Part model, mm, in its own coordinate system. Give positions to 0.01 mm unless a question says otherwise; leave off trailing zeros. Write item = value, one per line. Start each with the question number.
(1) Saw through at A-A, the plane y = 1.5. State how many separate pieces and enclosed holes the cut face has, then the cut area to 3 significant figures.
(2) Flat gauge pin, fed straight in: pin 1 (3 mm diameter, centred on x = 55.91, z = -55.35, fed in from -Y). Where does the tip first touch, or does it go through?
(3) Probe line 1 along X through (y, z) = (1.5, -90.5); line 2 along X through (y, z) = (0.25, 79.5). List the from-to ranges inside material, lowest first. Write a range as from..to.
from build123d import *

# Parameters (mm, degrees)
SKETCH1_W           = 482.6
SKETCH1_H           = 254
BOSS_EXTRUDE1_DEPTH = 3.175
FILLET1_R           = 6.35
CUT_EXTRUDE1_REACH  = 274.754
SKETCH3_R           = 3.05
CUT_EXTRUDE2_DEPTH  = 273.754491255
SKETCH4_R           = 2.5
CUT_EXTRUDE3_DEPTH  = 10


with BuildPart() as part:
    # Sketch1 → Boss-Extrude1 (new, symmetric)
    with BuildSketch(Plane(origin=(0, 0, 0), x_dir=(1, 0, 0), z_dir=(0, 1, 0))):
        Rectangle(SKETCH1_W, SKETCH1_H)
    extrude(amount=BOSS_EXTRUDE1_DEPTH, both=True)

    # Fillet1
    fillet1_edges = [part.edges().sort_by_distance(p)[0] for p in [
        (241.3, 0, 127),
        (-241.3, 0, 127),
        (-241.3, 0, -127),
        (241.3, 0, -127),
    ]]
    fillet(fillet1_edges, radius=FILLET1_R)

    # Sketch2 → Cut-Extrude1 (cut, up to next)
    with BuildSketch(Plane(origin=(0, 3.175, 0), x_dir=(1, 0, 0), z_dir=(0, 1, 0)), mode=Mode.PRIVATE) as cut_extrude1_sk1:
        with BuildLine():
            Line((227.25, -82.55), (227.25, -107.95))
            ThreePointArc((227.25, -107.95), (222.25, -112.95), (217.25, -107.95))
            Line((217.25, -107.95), (217.25, -82.55))
            ThreePointArc((217.25, -82.55), (222.25, -77.55), (227.25, -82.55))
        make_face()
    cut_extrude1_tool1 = extrude(cut_extrude1_sk1.sketch, amount=-CUT_EXTRUDE1_REACH, mode=Mode.PRIVATE) & part.part
    # Sketch2 → Cut-Extrude1 (cut, up to next)
    with BuildSketch(Plane(origin=(0, 3.175, 0), x_dir=(1, 0, 0), z_dir=(0, 1, 0)), mode=Mode.PRIVATE) as cut_extrude1_sk2:
        with BuildLine():
            Line((227.25, -44.45), (227.25, -19.05))
            ThreePointArc((227.25, -19.05), (222.25, -14.05), (217.25, -19.05))
            Line((217.25, -19.05), (217.25, -44.45))
            ThreePointArc((217.25, -44.45), (222.25, -49.45), (227.25, -44.45))
        make_face()
    cut_extrude1_tool2 = extrude(cut_extrude1_sk2.sketch, amount=-CUT_EXTRUDE1_REACH, mode=Mode.PRIVATE) & part.part
    # Sketch2 → Cut-Extrude1 (cut, up to next)
    with BuildSketch(Plane(origin=(0, 3.175, 0), x_dir=(1, 0, 0), z_dir=(0, 1, 0)), mode=Mode.PRIVATE) as cut_extrude1_sk3:
        with BuildLine():
            Line((227.25, 44.45), (227.25, 19.05))
            ThreePointArc((227.25, 19.05), (222.25, 14.05), (217.25, 19.05))
            Line((217.25, 19.05), (217.25, 44.45))
            ThreePointArc((217.25, 44.45), (222.25, 49.45), (227.25, 44.45))
        make_face()
    cut_extrude1_tool3 = extrude(cut_extrude1_sk3.sketch, amount=-CUT_EXTRUDE1_REACH, mode=Mode.PRIVATE) & part.part
    # Sketch2 → Cut-Extrude1 (cut, up to next)
    with BuildSketch(Plane(origin=(0, 3.175, 0), x_dir=(1, 0, 0), z_dir=(0, 1, 0)), mode=Mode.PRIVATE) as cut_extrude1_sk4:
        with BuildLine():
            Line((227.25, 82.55), (227.25, 107.95))
            ThreePointArc((227.25, 107.95), (222.25, 112.95), (217.25, 107.95))
            Line((217.25, 107.95), (217.25, 82.55))
            ThreePointArc((217.25, 82.55), (222.25, 77.55), (227.25, 82.55))
        make_face()
    cut_extrude1_tool4 = extrude(cut_extrude1_sk4.sketch, amount=-CUT_EXTRUDE1_REACH, mode=Mode.PRIVATE) & part.part
    # Sketch2 → Cut-Extrude1 (cut, up to next)
    with BuildSketch(Plane(origin=(0, 3.175, 0), x_dir=(1, 0, 0), z_dir=(0, 1, 0)), mode=Mode.PRIVATE) as cut_extrude1_sk5:
        with BuildLine():
            Line((-227.25, 82.55), (-227.25, 107.95))
            ThreePointArc((-227.25, 107.95), (-222.25, 112.95), (-217.25, 107.95))
            Line((-217.25, 107.95), (-217.25, 82.55))
            ThreePointArc((-217.25, 82.55), (-222.25, 77.55), (-227.25, 82.55))
        make_face()
    cut_extrude1_tool5 = extrude(cut_extrude1_sk5.sketch, amount=-CUT_EXTRUDE1_REACH, mode=Mode.PRIVATE) & part.part
    # Sketch2 → Cut-Extrude1 (cut, up to next)
    with BuildSketch(Plane(origin=(0, 3.175, 0), x_dir=(1, 0, 0), z_dir=(0, 1, 0)), mode=Mode.PRIVATE) as cut_extrude1_sk6:
        with BuildLine():
            Line((-227.25, 44.45), (-227.25, 19.05))
            ThreePointArc((-227.25, 19.05), (-222.25, 14.05), (-217.25, 19.05))
            Line((-217.25, 19.05), (-217.25, 44.45))
            ThreePointArc((-217.25, 44.45), (-222.25, 49.45), (-227.25, 44.45))
        make_face()
    cut_extrude1_tool6 = extrude(cut_extrude1_sk6.sketch, amount=-CUT_EXTRUDE1_REACH, mode=Mode.PRIVATE) & part.part
    # Sketch2 → Cut-Extrude1 (cut, up to next)
    with BuildSketch(Plane(origin=(0, 3.175, 0), x_dir=(1, 0, 0), z_dir=(0, 1, 0)), mode=Mode.PRIVATE) as cut_extrude1_sk7:
        with BuildLine():
            Line((-227.25, -44.45), (-227.25, -19.05))
            ThreePointArc((-227.25, -19.05), (-222.25, -14.05), (-217.25, -19.05))
            Line((-217.25, -19.05), (-217.25, -44.45))
            ThreePointArc((-217.25, -44.45), (-222.25, -49.45), (-227.25, -44.45))
        make_face()
    cut_extrude1_tool7 = extrude(cut_extrude1_sk7.sketch, amount=-CUT_EXTRUDE1_REACH, mode=Mode.PRIVATE) & part.part
    # Sketch2 → Cut-Extrude1 (cut, up to next)
    with BuildSketch(Plane(origin=(0, 3.175, 0), x_dir=(1, 0, 0), z_dir=(0, 1, 0)), mode=Mode.PRIVATE) as cut_extrude1_sk8:
        with BuildLine():
            Line((-227.25, -82.55), (-227.25, -107.95))
            ThreePointArc((-227.25, -107.95), (-222.25, -112.95), (-217.25, -107.95))
            Line((-217.25, -107.95), (-217.25, -82.55))
            ThreePointArc((-217.25, -82.55), (-222.25, -77.55), (-227.25, -82.55))
        make_face()
    cut_extrude1_tool8 = extrude(cut_extrude1_sk8.sketch, amount=-CUT_EXTRUDE1_REACH, mode=Mode.PRIVATE) & part.part
    add(cut_extrude1_tool1.solids().sort_by_distance((222.25, 3.175, 95.25))[0], mode=Mode.SUBTRACT)
    add(cut_extrude1_tool2.solids().sort_by_distance((222.25, 3.175, 31.75))[0], mode=Mode.SUBTRACT)
    add(cut_extrude1_tool3.solids().sort_by_distance((222.25, 3.175, -31.75))[0], mode=Mode.SUBTRACT)
    add(cut_extrude1_tool4.solids().sort_by_distance((222.25, 3.175, -95.25))[0], mode=Mode.SUBTRACT)
    add(cut_extrude1_tool5.solids().sort_by_distance((-222.25, 3.175, -95.25))[0], mode=Mode.SUBTRACT)
    add(cut_extrude1_tool6.solids().sort_by_distance((-222.25, 3.175, -31.75))[0], mode=Mode.SUBTRACT)
    add(cut_extrude1_tool7.solids().sort_by_distance((-222.25, 3.175, 31.75))[0], mode=Mode.SUBTRACT)
    add(cut_extrude1_tool8.solids().sort_by_distance((-222.25, 3.175, 95.25))[0], mode=Mode.SUBTRACT)

    # Sketch3 → Cut-Extrude2 (cut, through all)
    with BuildSketch(Plane(origin=(0, 3.175, 0), x_dir=(1, 0, 0), z_dir=(0, 1, 0))):
        with Locations(Location((-50.8, 98.955999998, 0), (0, 0, 270))):
            Circle(SKETCH3_R)
        with Locations(Location((-50.8, 63.955999998, 0), (0, 0, 270))):
            Circle(SKETCH3_R)
        with Locations(Location((-50.8, 28.955999998, 0), (0, 0, 270))):
            Circle(SKETCH3_R)
    extrude(amount=-CUT_EXTRUDE2_DEPTH, mode=Mode.SUBTRACT)

    # Sketch4 → Cut-Extrude3 (cut)
    with BuildSketch(Plane.XZ.offset(-3.175)):
        with Locations(Location((55.899172715, 20.049660002, 0), (0, 0, 90))):
            Circle(SKETCH4_R)
        with Locations(Location((-9.929521758, 20.049660002, 0), (0, 0, 90))):
            Circle(SKETCH4_R)
        with Locations(Location((55.912941777, -55.350339998, 0), (0, 0, 90))):
            Circle(SKETCH4_R)
        with Locations(Location((-9.943351442, -55.363639998, 0), (0, 0, 90))):
            Circle(SKETCH4_R)
    extrude(amount=CUT_EXTRUDE3_DEPTH, mode=Mode.SUBTRACT)


solid = part.part
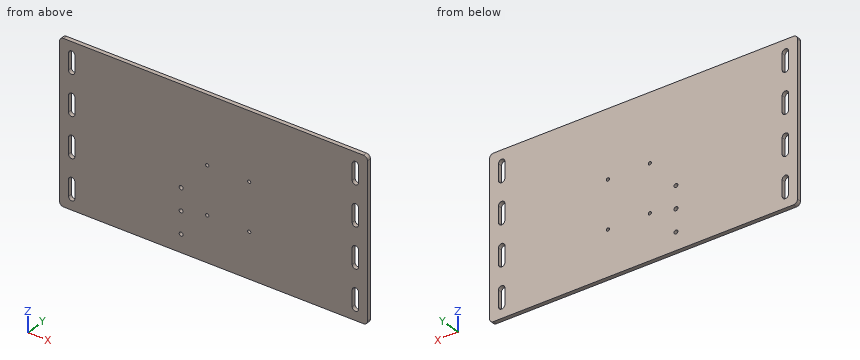
Results list:
q1.separate_pieces = 1
q1.enclosed_holes = 15
q1.area = 120,000 mm^2
q2.pin_1 = through
q3.line_1 = -241.3..-227.25, -217.25..217.25, 227.25..241.3
q3.line_2 = -241.3..-226.21, -218.29..218.29, 226.21..241.3
